```python
from build123d import *

# Parameters (mm, degrees)
SKETCH003_W     = 130
SKETCH003_H     = 165
PAD002_DEPTH    = 6
SKETCH004_W     = 120
SKETCH004_H     = 155
POCKET001_DEPTH = 10
SKETCH007_W     = 130
SKETCH007_H     = 165
SKETCH007_W_2   = 124.9
SKETCH007_H_2   = 159.9
POCKET002_DEPTH = 2
SKETCH008_R     = 4
PAD004_DEPTH    = 6
SKETCH009_R     = 3.1
POCKET003_DEPTH = 3.2
FILLET001_R     = 2
FILLET002_R     = 1
FILLET003_R     = 1
FILLET004_R     = 1
FILLET005_R     = 1


with BuildPart() as part:
    # Sketch003 → Pad002 (new body)
    with BuildSketch(Plane.XY):
        Rectangle(SKETCH003_W, SKETCH003_H)
    extrude(amount=PAD002_DEPTH)

    # Sketch004 (on Face6 of Pad002) → Pocket001 (cut)
    with BuildSketch(Plane.XY.offset(6)):
        Rectangle(SKETCH004_W, SKETCH004_H)
    extrude(amount=-POCKET001_DEPTH, mode=Mode.SUBTRACT)

    # Sketch007 (on Face5 of Pocket001) → Pocket002 (cut)
    with BuildSketch(Plane.XY.offset(6)):
        Rectangle(SKETCH007_W, SKETCH007_H)
        Rectangle(SKETCH007_W_2, SKETCH007_H_2, mode=Mode.SUBTRACT)
    extrude(amount=-POCKET002_DEPTH, mode=Mode.SUBTRACT)

    # Sketch008 (on Face2 of Pocket002) → Pad004 (join)
    with BuildSketch(Plane(origin=(0, 0, 0), x_dir=(1, 0, 0), z_dir=(0, 0, -1))):
        with Locations((-56.877501, 75)):
            Circle(SKETCH008_R)
        with Locations((56.877501, 75)):
            Circle(SKETCH008_R)
        with Locations((-56.877501, -75)):
            Circle(SKETCH008_R)
        with Locations((56.877501, -75)):
            Circle(SKETCH008_R)
    extrude(amount=-PAD004_DEPTH)

    # Sketch009 (on Face10 of Pad004) → Pocket003 (cut)
    with BuildSketch(Plane(origin=(0, 0, 0), x_dir=(1, 0, 0), z_dir=(0, 0, -1))):
        with Locations((-56.877501, 75)):
            Circle(SKETCH009_R)
        with Locations((56.877501, 75)):
            Circle(SKETCH009_R)
        with Locations((-56.877501, -75)):
            Circle(SKETCH009_R)
        with Locations((56.877501, -75)):
            Circle(SKETCH009_R)
    extrude(amount=-POCKET003_DEPTH, mode=Mode.SUBTRACT)

    # Fillet001
    fillet001_edges = [part.edges().sort_by_distance(p)[0] for p in [
        (65, -82.5, 2),
        (-65, -82.5, 2),
        (-65, 82.5, 2),
        (65, 82.5, 2),
    ]]
    fillet(fillet001_edges, radius=FILLET001_R)

    # Fillet002
    fillet002_edges = [part.edges().sort_by_distance(p)[0] for p in [
        (62.45, -79.95, 5),
    ]]
    fillet(fillet002_edges, radius=FILLET002_R)

    # Fillet003
    fillet003_edges = [part.edges().sort_by_distance(p)[0] for p in [
        (-62.45, -79.95, 5),
    ]]
    fillet(fillet003_edges, radius=FILLET003_R)

    # Fillet004
    fillet004_edges = [part.edges().sort_by_distance(p)[0] for p in [
        (-62.45, 79.95, 5),
    ]]
    fillet(fillet004_edges, radius=FILLET004_R)

    # Fillet005
    fillet005_edges = [part.edges().sort_by_distance(p)[0] for p in [
        (62.45, 79.95, 5),
    ]]
    fillet(fillet005_edges, radius=FILLET005_R)


solid = part.part
```
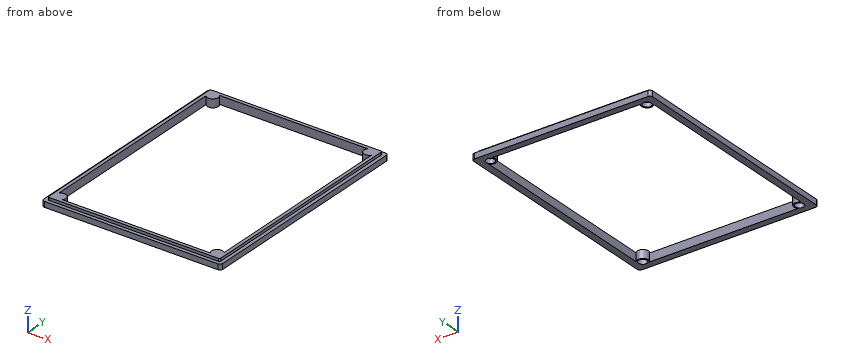
Could you check a few things on this model? Use its own coordinates, in mm. Coordinates: 2 decimals unless noted, no trailing zeros. Order: outer loops, then holes, each group sorted by start corner. A loop starts at its lowest first (then second) coordinate and runs counter-clockwise, first axis right, second up. Notation, with made-up numbers: M 42.25,6.25 L 47.25,6.25 A30 cw 47.25,28.25 Z; hole C 8,-34.75 d2. An arc over 180 degrees is marked long. Use one line per item in the form item = value. Start each with the question number.
1. Suppose I cut it at B-B on y = 75. Write out the boundary of the cut face in (x, z).
2. Suppose I cut it at C-C on z = 1.6. Write out the boundary of the cut face in (x, y) (1 decimal).
3. Please list where these lines run through material, in increasing order: line 1 (X direction, y = 75, z = 1.1); line 2 (Y direction, x = 47.5, z = 1.6); line 3 (X direction, y = -51, z = 2).
4. For pin 1 (1.9 mm diameter, centred on x = 56.5, y = 75.5, fed in from -Z); pin 2 (0.6 mm diameter, centred on y = -17.5, z = 5, fed in from -X); pin 3 (1.6 mm diameter, centred on y = -38.5, z = 5, fed in from +X), each with a flat end and sliding along its axis, tell me the tip position at first contact or that it passes through.
5. Suppose I cut it at A-A on x = 28. Write out the boundary of the cut face in (y, z), then the cut area to 3 significant figures.
6. Suppose I cut it at D-D on y = -36. Write out the boundary of the cut face in (x, z).
Geometry says:
q1.outline = M -65,0 L -59.98,0 L -59.98,3.2 L -53.78,3.2 L -53.78,0 L -52.88,0 L -52.88,6 L -62.45,6 L -62.45,4 L -65,4 Z; M 52.88,0 L 53.78,0 L 53.78,3.2 L 59.98,3.2 L 59.98,0 L 65,0 L 65,4 L 62.45,4 L 62.45,6 L 52.88,6 Z
q2.outline = M -65,-80.5 A2 ccw -63,-82.5 L 63,-82.5 A2 ccw 65,-80.5 L 65,80.5 A2 ccw 63,82.5 L -63,82.5 A2 ccw -65,80.5 Z; hole C -56.9,-75 d6.2; hole M -60,-72.5 A4 cw -53.8,-77.5 L 53.8,-77.5 A4 cw 60,-72.5 L 60,72.5 A4 cw 53.8,77.5 L -53.8,77.5 A4 cw -60,72.5 Z; hole C -56.9,75 d6.2; hole C 56.9,-75 d6.2; hole C 56.9,75 d6.2
q3.line_1 = -65 to -59.98, -53.78 to -52.88, 52.88 to 53.78, 59.98 to 65
q3.line_2 = -82.5 to -77.5, 77.5 to 82.5
q3.line_3 = -65 to -60, 60 to 65
q4.pin_1 = 3.2
q4.pin_2 = -62.45
q4.pin_3 = 62.45
q5.outline = M -82.5,0 L -77.5,0 L -77.5,6 L -79.95,6 L -79.95,4 L -82.5,4 Z; M 77.5,0 L 82.5,0 L 82.5,4 L 79.95,4 L 79.95,6 L 77.5,6 Z
q5.area = 49.8 mm^2
q6.outline = M -65,0 L -60,0 L -60,6 L -62.45,6 L -62.45,4 L -65,4 Z; M 60,0 L 65,0 L 65,4 L 62.45,4 L 62.45,6 L 60,6 Z
